Here's how the part is built. I have some questions about the finished solid (model axes, mm). A direction names the side the tool comes from. Round coordinates to 2 decimals unless told otherwise and drop trailing zeros. Write each loop counter-clockwise with the first axis right and the second up, starting at its lowest first coordinate (ties: lowest second). Pieces come first, ordered by that corner, then holes. Notation, with made-up numbers: (-10.75, 84) -> (3.25, 84) arc R22 ccw to (3.25, 93) -> close; hole circle Ø7 at (80, -1). An arc over 180 degrees is marked (long way). Put each result on its own line as item: value. Start each with the question number.
1) I want a section at D-D, the plane z = -3.25. List the corners of the cut face in (x, y) for me.
2) If I drill on line 1 along X through (y, z) = (2, -0.75); line 2 along Z through (x, y) = (7.5, 0.5); line 3 along Z through (x, y) = (15, 2), over which ranges is the centre line in solid material (lowest first)? Write a range as [from, to].
3) We'd pull the mould along Z, two halves only. Please class faces 3 (the flat face through (16, -2, -2)), 4 (the cylindrical face through (0.49, -4.88, 1.08)), 5 (the flat face through (9, -1, 2)): released by +Z, released by -Z, zero draft, split by the parting line, or undercut.
4) Will these pins go through, and if not, where does the flat tip stop? P1, Ø6, axis at x = 10, y = -3, coming from the -Z side; P2, Ø6, axis at x = 14, z = 3, coming from the -Y side; P3, Ø1.6, axis at x = 9.5, z = -2, coming from the -Y side.
5) I want a section at B-B, the plane x = 8.25. List the corners of the cut face in (y, z) for me.
6) I want a section at A-A, the plane z = 0. List the corners of the cut face in (x, y) for me.
7) Which directions (+Z, -Z, +X, -X, +Y, -Y) give clear straight access to the entire face, cutting with the end or side of a thin tool? Please do faces 1 (the flat face through (0, 0, 0)), 2 (the flat face through (9, 2, -1)).
from build123d import *

# Parameters (mm, degrees)
SKETCH1_R           = 5
BOSS_EXTRUDE2_DEPTH = 1
SKETCH2_R           = 4
BOSS_EXTRUDE3_DEPTH = 15
CUT_EXTRUDE1_DEPTH  = 15


with BuildPart() as part:
    # Sketch1 → Boss-Extrude2 (new body)
    with BuildSketch(Plane(origin=(0, 0, 0), x_dir=(0, 0, -1), z_dir=(1, 0, 0))):
        Circle(SKETCH1_R)
    extrude(amount=BOSS_EXTRUDE2_DEPTH)

    # Sketch2 → Boss-Extrude3 (add)
    with BuildSketch(Plane(origin=(1, 0, 0), x_dir=(0, 0, -1), z_dir=(1, 0, 0))):
        Circle(SKETCH2_R)
    extrude(amount=BOSS_EXTRUDE3_DEPTH)

    # Sketch4 → Cut-Extrude1 (cut)
    with BuildSketch(Plane(origin=(16, 0, 0), x_dir=(0, 0, -1), z_dir=(1, 0, 0))):
        Polygon((1, 2.5), (0, 2.5), (-1, 2.5), (-1, 1), (0, 1), (1, 1), align=None)
        Polygon((0, 1), (-1, 1), (-1, 0), (-1, -1), (-0.604082815, -1), (1, -1), (1, 0), (1, 1), align=None)
        Polygon((2.5, 1), (1, 1), (1, 0), (1, -1), (2.5, -1), (2.5, 0), align=None)
        Polygon((-1, 0), (-1, 1), (-2.5, 1), (-2.5, 0), (-2.5, -1), (-1, -1), align=None)
        Polygon((-0.604082815, -1), (-1, -1), (-1, -2.5), (-0.604082815, -2.5), (1, -2.5), (1, -1), align=None)
    extrude(amount=-CUT_EXTRUDE1_DEPTH, mode=Mode.SUBTRACT)


solid = part.part
Findings:
1. outline: (0, -3.8) -> (1, -3.8) -> (1, -2.33) -> (16, -2.33) -> (16, 2.33) -> (1, 2.33) -> (1, 3.8) -> (0, 3.8) -> close
2. line 1: x = [0, 1]
2. line 2: z = [-3.97, -2.5], [2.5, 3.97]
2. line 3: z = [-3.46, -1], [1, 3.46]
3. face 3: zero draft
3. face 4: split by the parting line
3. face 5: undercut
4. P1: stops at z = -4
4. P2: stops at y = -4
4. P3: stops at y = -3.82
5. outline: circle Ø8 at (0, 0); hole (-2.5, -1) -> (-1, -1) -> (-1, -2.5) -> (1, -2.5) -> (1, -1) -> (2.5, -1) -> (2.5, 1) -> (1, 1) -> (1, 2.5) -> (-1, 2.5) -> (-1, 1) -> (-2.5, 1) -> close
6. outline: (0, -5) -> (1, -5) -> (1, -4) -> (16, -4) -> (16, -2.5) -> (1, -2.5) -> (1, 2.5) -> (16, 2.5) -> (16, 4) -> (1, 4) -> (1, 5) -> (0, 5) -> close
7. face 1: +Z, -Z, -X, +Y, -Y
7. face 2: +X
